from build123d import *

# Parameters (mm, degrees)
F1_DEPTH = 25.4
F2_DEPTH = 50.8
F3_DEPTH = 9.525
F5_R     = 6.35


with BuildPart() as f1:
    # F0 (on Front) → F1 (new body, symmetric)
    with BuildSketch(Plane.XZ):
        Polygon((86.0920930787, 65.0018583123), (60.325, 65.0018583123), (60.325, 45.9518583123), (85.8321436333, 45.9518583123), align=None)
        with BuildLine():
            Line((22.225, 9.525), (41.275, 9.525))
            Line((41.275, 9.525), (41.275, 30.1144513303))
            ThreePointArc((41.275, 30.1144513303), (46.3175880369, 41.7193845943), (58.2418631259, 45.9518583123))
            Line((58.2418631259, 45.9518583123), (60.325, 45.9518583123))
            Line((60.325, 45.9518583123), (60.325, 65.0018583123))
            Line((60.325, 65.0018583123), (55.5299817685, 65.0018583123))
            ThreePointArc((55.5299817685, 65.0018583123), (31.8880250006, 54.2305920691), (22.225, 30.1144513303))
            Line((22.225, 30.1144513303), (22.225, 9.525))
        make_face()
    extrude(amount=F1_DEPTH, both=True)

    # F0 (on Front) → F2 (join, symmetric)
    with BuildSketch(Plane.XZ):
        Polygon((-41.275, 9.525), (-41.275, -9.525), (41.275, -9.525), (41.275, 9.525), (22.225, 9.525), align=None)
    extrude(amount=F2_DEPTH, both=True)

    # F0 (on Front) → F3 (join, symmetric)
    with BuildSketch(Plane.XZ):
        with BuildLine():
            add(Edge.make_bspline(
                [(55.5299817685, 65.0018583123), (17.2289203086, 64.6301832149), (-41.1762930453, 21.5798933059), (-41.275, 9.525)],
                knots=[0, 0, 0, 0, 111.5745773167, 111.5745773167, 111.5745773167, 111.5745773167], degree=3))
            Line((-41.275, 9.525), (22.225, 9.525))
            Line((22.225, 9.525), (22.225, 30.1144513303))
            ThreePointArc((22.225, 30.1144513303), (31.8880250006, 54.2305920691), (55.5299817685, 65.0018583123))
        make_face()
    extrude(amount=F3_DEPTH, both=True)

    # F0 (on Front) → F4 (revolve)
    with BuildSketch(Plane.XZ):
        Polygon((86.1149241681, 66.675), (86.0920930787, 65.0018583123), (85.8321436333, 45.9518583123), (85.725, 38.1), (111.125, 38.1), (111.125, 66.675), align=None)
    revolve(axis=Axis((85.9199620841, 0, 52.3875), (0.0136443699, 0, 0.9999069113)))

    # F5
    f5_edges = [f1.edges().sort_by_distance(p)[0] for p in [
        (41.275, -50.8, 0),
        (-41.275, -50.8, 0),
        (41.275, 50.8, 0),
        (-41.275, 50.8, 0),
    ]]
    fillet(f5_edges, radius=F5_R)


solid = f1.part
Model file for the job. Use its own axes, mm. A direction names the side the tool comes from. Round coordinates to 2 decimals unless told otherwise and drop trailing zeros. Order: outer loops, then holes, each group sorted by start corner. A loop starts at its lowest first (then second) coordinate and runs counter-clockwise, first axis right, second up.
(1) Pin check, flat tips, straight feed: pin 1 (6 mm diameter, centred on y = -3.5, z = 8, fed in from +X) (3 decimals); pin 2 (10 mm diameter, centred on x = 69.5, y = -6.5, fed in from -Z); pin 3 (8 mm diameter, centred on y = 7.5, z = 35, fed in from +X); pin 4 (17.5 mm diameter, centred on y = -16.5, z = 16.5, fed in from -X) (3 decimals). Stop position of each tip, or through.
(2) Drill centre lines: line 1 (Z direction, x = -27.5, y = 37.5) (3 decimals); line 2 (X direction, y = 5.5, z = 0.5) (3 decimals). Where is each one in solid material? Low to high.
(3) 3-axis set-ups, long thin cutter, end or side, ignore diameter. For faces 4 (the face through (60.7, -0.1, 65.002)), 5 (the face through (32.15, 17.35, 54.5)), 6 (the face through (3, -9.525, 29)), 7 (the face through (41.275, -1, 6)): which of +Z, -Z, +X, -X, +Y, -Y reach the whole face in a straight line?
(4) Pull direction X, two halves, no side cores. Call faces 1 (the face through (1, -30, 9.525)), 2 (the face through (60, -2, 45.952)), 3 (the face through (22.225, -18, 20)): released by +X, released by -X, zero draft, split by the parting line, or undercut.
(5) Band-saw the part on A-A (y = -31). List the corners of the cut face in (x, z) (3 decimals), then the cut area to 3 significant figures.
Verdict:
1. pin 1: stops at x = 41.275
1. pin 2: stops at z = 38.43
1. pin 3: stops at x = 110.63
1. pin 4: stops at x = -41.275
2. line 1: z = -9.525 to 9.525
2. line 2: x = -41.275 to 41.275
3. face 4: +Z, -X
3. face 5: +Z, -X, +Y
3. face 6: +Z, -X, -Y
3. face 7: -Z, +X, +Y, -Y
4. face 1: zero draft
4. face 2: undercut
4. face 3: released by -X
5. outline: (-41.275, -9.525) - (41.275, -9.525) - (41.275, 9.525) - (-41.275, 9.525) - close
5. area: 1,570 mm2
